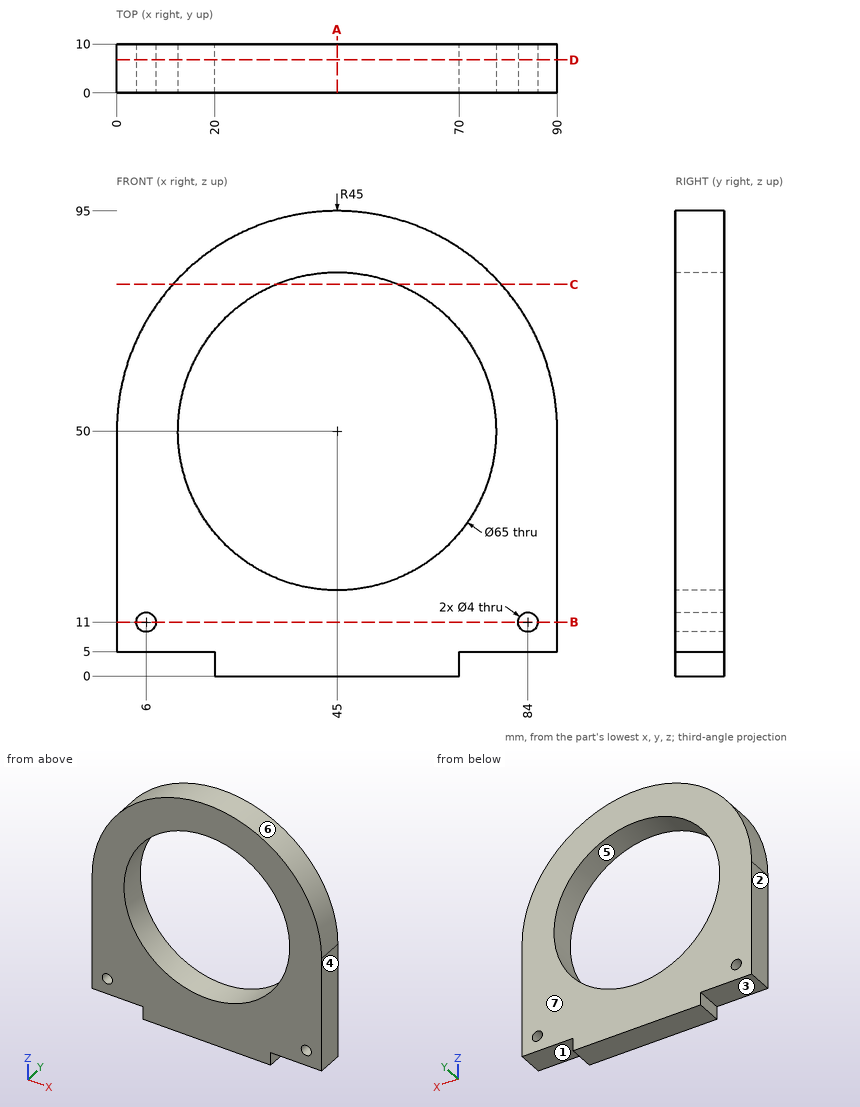
Could you check a few things on this drawing? It's one solid part, dimensions in mm from its lowest x, y, z. A direction names the side the tool comes from. Give positions to 0.01 mm unless a question says otherwise; leave off trailing zeros. Order: outer loops, then holes, each group sorted by start corner. A loop starts at its lowest first (then second) coordinate and runs counter-clockwise, first axis right, second up.
1. Suppose I cut it at D-D (y = 6.75). Write out the boundary of the cut face in (x, z).
Answers below:
outline: (0, 5) - (20, 5) - (20, 0) - (70, 0) - (70, 5) - (90, 5) - (90, 50) arc R45 ccw to (0, 50) - close; hole circle Ø4 at (6, 11); hole circle Ø65 at (45, 50); hole circle Ø4 at (84, 11)
2. I need wall thicknesses on L1, parallel to X at y = 3, z = 11; L2, parallel to X at y = 5.5, z = 50; L3, parallel to Z at x = 44.5, y = 7.75. Which ranges of each line are inside material? Lowest first, please.
Answers below:
L1: x = 0 to 4, 8 to 82, 86 to 90
L2: x = 0 to 12.5, 77.5 to 90
L3: z = 0 to 17.5, 82.5 to 95
3. Which directions (+Z, -Z, +X, -X, +Y, -Y) give clear straight access to the entire face, cutting with the end or side of a thin tool? Please do the marked faces 1, 2 and 3.
Answers below:
face 1: -Z, +X, +Y, -Y
face 2: +Z, -Z, -X, +Y, -Y
face 3: -Z, -X, +Y, -Y
4. Suppose I cut it at A-A (x = 45). Write out the boundary of the cut face in (y, z), plus the area to 3 significant figures.
Answers below:
outline: (0, 0) - (10, 0) - (10, 17.5) - (0, 17.5) - close; (0, 82.5) - (10, 82.5) - (10, 95) - (0, 95) - close
area: 300 mm2
5. Suppose I cut it at B-B (z = 11). Write out the boundary of the cut face in (x, y), plus the area to 3 significant figures.
Answers below:
outline: (0, 0) - (4, 0) - (4, 10) - (0, 10) - close; (8, 0) - (82, 0) - (82, 10) - (8, 10) - close; (86, 0) - (90, 0) - (90, 10) - (86, 10) - close
area: 820 mm2
6. Suppose I cut it at C-C (z = 80). Write out the boundary of the cut face in (x, y), plus the area to 3 significant figures.
Answers below:
outline: (11.46, 0) - (32.5, 0) - (32.5, 10) - (11.46, 10) - close; (57.5, 0) - (78.54, 0) - (78.54, 10) - (57.5, 10) - close
area: 421 mm2
7. For pin 1 (6 mm diameter, centred on y = 4.5, z = 71, fed in from -X); pin 2 (2.5 mm diameter, centred on y = 6.5, z = 3.5, fed in from -X); pin 3 (1 mm diameter, centred on y = 3.5, z = 51.5, fed in from +X), each with a flat end and sliding along its axis, tell me the tip position at first contact or that it passes through.
Answers below:
pin 1: stops at x = 3.76
pin 2: stops at x = 20
pin 3: stops at x = 89.99
8. Thinking about a two-plate mould opening in X: for the marked faces 4, 5, 6 and 7, which applies, +X half, -X half, draft (parallel to the pull), parting line (faces both ways), or undercut?
Answers below:
face 4: +X half
face 5: undercut
face 6: parting line
face 7: draft
